from build123d import *

# Parameters (mm, degrees)
SKETCH_W     = 64
SKETCH_H     = 5
PAD_DEPTH    = 2
SKETCH001_W  = 3
SKETCH001_H  = 5
PAD001_DEPTH = 5.5
SKETCH003_W  = 3
SKETCH003_H  = 5
PAD002_DEPTH = 10
SKETCH004_R  = 0.75
POCKET_DEPTH = 100
FILLET_R     = 2.49


with BuildPart() as part:
    # Sketch → Pad (new body)
    with BuildSketch(Plane.XY):
        Rectangle(SKETCH_W, SKETCH_H)
    extrude(amount=PAD_DEPTH)

    # Sketch001 (on Face6 of Pad) → Pad001 (join)
    with BuildSketch(Plane.XY.offset(2)):
        with Locations((-30.5, 0)):
            Rectangle(SKETCH001_W, SKETCH001_H)
        with Locations((30.5, 0)):
            Rectangle(SKETCH001_W, SKETCH001_H)
    extrude(amount=PAD001_DEPTH)

    # Sketch003 → Pad002 (join)
    with BuildSketch(Plane(origin=(0, 0, 0), x_dir=(1, 0, 0), z_dir=(0, 0, -1))):
        with Locations((-27.3, 0)):
            Rectangle(SKETCH003_W, SKETCH003_H)
        with Locations((27.3, 0)):
            Rectangle(SKETCH003_W, SKETCH003_H)
    extrude(amount=PAD002_DEPTH)

    # Sketch004 (on Face13 of Pad002) → Pocket (cut)
    with BuildSketch(Plane(origin=(-32, 0, 0), x_dir=(0, -1, 0), z_dir=(-1, 0, 0))):
        with Locations((0, 5)):
            Circle(SKETCH004_R)
    extrude(amount=-POCKET_DEPTH, mode=Mode.SUBTRACT)

    # Fillet
    fillet_edges = [part.edges().sort_by_distance(p)[0] for p in [
        (30.5, -2.5, 7.5),
        (30.5, 2.5, 7.5),
        (-30.5, -2.5, 7.5),
        (-30.5, 2.5, 7.5),
    ]]
    fillet(fillet_edges, radius=FILLET_R)


solid = part.part
Build history of the part. All positions in model axes, mm. A direction names the side the tool comes from. Round coordinates to 2 decimals unless told otherwise and drop trailing zeros. Write each loop counter-clockwise with the first axis right and the second up, starting at its lowest first coordinate (ties: lowest second). Pieces come first, ordered by that corner, then holes. Notation, with made-up numbers: M -40,-2 L 16,-2 A38 cw 16,37 Z; hole C 10,54.5 d4. An arc over 180 degrees is marked long. Answer as a JSON object with one key per item and string values. Group by question number.
(1) Cut at C-C (x = 27). Give the cut face in (y, z), and give its area (3 significant figures).
(2) Which spindle directions (+Z, -Z, +X, -X, +Y, -Y) get a long thin tool onto all of the face, cutting with end or side? Do faces 4 (the flat face through (0, 0, 0)), 5 (the cylindrical face through (-30.48, 1.75, 6.79)), 6 (the flat face through (-30, 0, 0)), 7 (the flat face through (29, 0, 4)), 8 (the flat face through (30, 0, 0)). Say none if no direction does.
(3) Mould opens along Y. For faces 1 (the flat face through (27, 0, -10)), 2 (the cylindrical face through (30.52, -1.79, 6.75)), 3 (the cylindrical face through (30.479, 0.163, 4.268)) say: pulls with the +Y half, pulls with the -Y half, needs draft (parallel to the pull), parting line crosses it, or undercut.
(4) Flat gauge pins, fed straight in: pin 1 (2.5 mm diameter, centred on x = 30.5, y = -1, fed in from -Z); pin 2 (1 mm diameter, centred on x = 13, z = -1, fed in from +Y); pin 3 (2.5 mm diameter, centred on y = 0.5, z = -3.5, fed in from +X); pin 4 (2.5 mm diameter, centred on x = 11.5, y = 1, fed in from +Z). Where does each tip first touch, or does it go through?
(5) Cut at B-B (x = -8.5). Give the cut face in (y, z), and give its area (3 significant figures).
(6) Cut at A-A (y = 1.3). Give the cut face in (x, z).
(7) Drill centre lines: L1, parallel to Z at x = -30.95, y = 0; L2, parallel to X at y = 1.8, z = 3.75; L3, parallel to X at y = 1.95, z = -2. Where is each one in solid material? Low to high.
Responses:
{
 "1": {"outline": "M -2.5,-10 L 2.5,-10 L 2.5,2 L -2.5,2 Z", "area": "60.0 mm2"},
 "2": {"face 4": "-Z, +Y, -Y", "face 5": "+Z, +X, -X, +Y", "face 6": "-Z, -X, +Y, -Y", "face 7": "+Z, +Y, -Y", "face 8": "-Z, +X, +Y, -Y"},
 "3": {"face 1": "needs draft", "face 2": "pulls with the -Y half", "face 3": "undercut"},
 "4": {"pin 1": "stops at z = 0", "pin 2": "passes through", "pin 3": "stops at x = 28.8", "pin 4": "stops at z = 2"},
 "5": {"outline": "M -2.5,0 L 2.5,0 L 2.5,2 L -2.5,2 Z", "area": "10.0 mm2"},
 "6": {"outline": "M -32,0 L -28.8,0 L -28.8,-10 L -25.8,-10 L -25.8,0 L 25.8,0 L 25.8,-10 L 28.8,-10 L 28.8,0 L 32,0 L 32,7.14 L 29,7.14 L 29,2 L -29,2 L -29,7.14 L -32,7.14 Z"},
 "7": {"L1": "z = 0 to 4.25, 5.75 to 7.5", "L2": "x = -32 to -29, 29 to 32", "L3": "x = -28.8 to -25.8, 25.8 to 28.8"}
}
